Part model, mm, in its own coordinate system. Face numbers are marked on the shaded views. A direction names the side the tool comes from. Round coordinates to 2 decimals unless told otherwise and drop trailing zeros. Order: outer loops, then holes, each group sorted by start corner. A loop starts at its lowest first (then second) coordinate and runs counter-clockwise, first axis right, second up. Notation, with made-up numbers: M 15,21 L 56,21 A32 cw 56,60 Z; hole C -18.75,-22.5 d3. An arc over 180 degrees is marked long. One line per question, with ' | ' between items.
from build123d import *

# Parameters (mm, degrees)
F1_DEPTH = 20
F3_DEPTH = 25
F4_R     = 0.25


with BuildPart() as f1:
    # F0 (on Top) → F1 (new body)
    with BuildSketch(Plane.XY):
        Polygon((-10, 8.5), (-10, 3.75), (-8.75, 3.75), (-8.75, -3.75), (-10, -3.75), (-10, -8.5), (-2.5, -8.5), (-2.5, -3.75), (-3.75, -3.75), (-3.75, 0), (2.5, -8.5), (10, -8.5), (10, -3.75), (8.75, -3.75), (8.75, 3.75), (10, 3.75), (10, 8.5), (2.5, 8.5), (2.5, 3.75), (3.75, 3.75), (3.75, 0), (-2.5, 8.5), align=None)
    extrude(amount=F1_DEPTH)

    # F2 (on face) → F3 (cut)
    with BuildSketch(Plane.XY.offset(20)):
        with BuildLine():
            ThreePointArc((-8.422959, 7.125), (-8.797959, 7.5), (-9.172959, 7.125))
            Line((-9.172959, 7.125), (-9.172959, 5.125))
            ThreePointArc((-9.172959, 5.125), (-8.797959, 4.75), (-8.422959, 5.125))
            Line((-8.422959, 5.125), (-8.422959, 7.125))
        make_face()
    extrude(amount=-F3_DEPTH, mode=Mode.SUBTRACT)

    # F4
    f4_edges = [f1.edges().sort_by_distance(p)[0] for p in [
        (-10, 8.5, 10),
        (2.5, 8.5, 10),
        (-2.5, 8.5, 10),
        (2.5, 3.75, 10),
        (10, 3.75, 10),
        (10, 8.5, 10),
        (10, -3.75, 10),
        (10, -8.5, 10),
        (2.5, -8.5, 10),
        (-2.5, -3.75, 10),
        (-2.5, -8.5, 10),
        (-10, -8.5, 10),
        (-10, -3.75, 10),
        (-8.75, -3.75, 10),
        (-3.75, -3.75, 10),
        (-8.75, 3.75, 10),
        (-10, 3.75, 10),
        (3.75, 3.75, 10),
        (8.75, 3.75, 10),
        (8.75, -3.75, 10),
    ]]
    fillet(f4_edges, radius=F4_R)


solid = f1.part
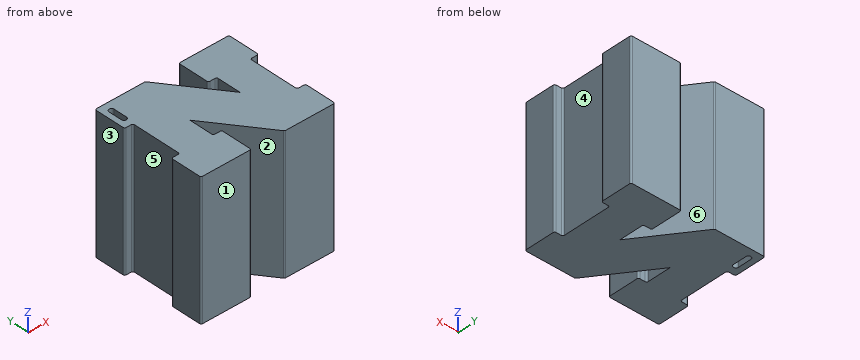
1) Saw through at D-D (y = -2.75). List the corners of the cut face in (x, z), plus the area to 3 significant figures.
The answers:
outline: M -8.75,0 L -3.75,0 L -3.75,20 L -8.75,20 Z; M -1.73,0 L 8.75,0 L 8.75,20 L -1.73,20 Z | area: 310 mm²
2) Which spindle directions (+Z, -Z, +X, -X, +Y, -Y) get a long thin tool onto all of the face, cutting with end or side? Do the marked faces 4, 5 and 6. Say none if no direction does.
The answers:
face 4: +Z, -Z, +X | face 5: +Z, -Z, -X | face 6: +Z, -Z
3) Drop flat-ended pins along their axis: pin 1 (6 mm diameter, centred on y = -0.5, z = 16.5, fed in from +X); pin 2 (2 mm diameter, centred on x = 1.5, z = 6.5, fed in from -Y); pin 3 (1.8 mm diameter, centred on y = 1, z = 8.5, fed in from -X). Give the stop position or say it passes through.
The answers:
pin 1: stops at x = 8.75 | pin 2: stops at y = -8.47 | pin 3: stops at x = -8.75
4) Saw through at A-A (y = -6.25). List the corners of the cut face in (x, z), plus the area to 3 significant figures.
The answers:
outline: M -10,0 L -2.5,0 L -2.5,20 L -10,20 Z; M 0.85,0 L 10,0 L 10,20 L 0.85,20 Z | area: 333 mm²
5) Probe line 1 (X direction, y = 5, z = 14); line 2 (X direction, y = 6, z = 14.5); line 3 (Y direction, x = 9, z = 8). List the from-to ranges inside material, lowest first. Write a range as [from, to].
The answers:
line 1: x = [-10, -9.15], [-8.44, 0.07], [2.5, 10] | line 2: x = [-10, -9.17], [-8.42, -0.66], [2.5, 10] | line 3: y = [-8.5, -3.75], [3.75, 8.5]
6) Saw through at B-B (y = 5.75). List the corners of the cut face in (x, z), plus the area to 3 significant figures.
The answers:
outline: M -10,0 L -9.17,0 L -9.17,20 L -10,20 Z; M -8.42,0 L -0.48,0 L -0.48,20 L -8.42,20 Z; M 2.5,0 L 10,0 L 10,20 L 2.5,20 Z | area: 325 mm²
7) Saw through at C-C (x = 0.75). List the corners of the cut face in (y, z), plus the area to 3 significant figures.
The answers:
outline: M -6.12,0 L 4.08,0 L 4.08,20 L -6.12,20 Z | area: 204 mm²
8) Two-plate mould, pull along Y, no slides. Class the marked faces 1, 2 and 3: released by +Y, released by -Y, zero draft, split by the parting line, or undercut.
The answers:
face 1: released by -Y | face 2: undercut | face 3: zero draft
